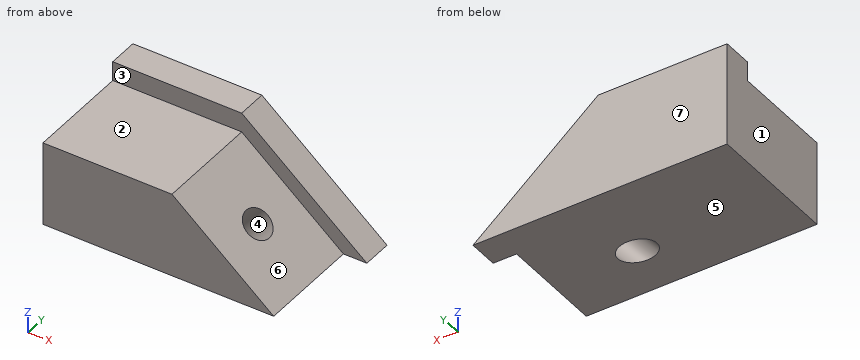
from build123d import *

# Parameters (mm, degrees)
F0_W     = 126.0763704777
F0_H     = 65.8090934157
F1_DEPTH = 50.8
F3_DEPTH = 51.054
F5_DEPTH = 25.4
F6_R     = 7.3849812588
F7_DEPTH = 47.244


with BuildPart() as f1:
    # F0 (on Top) → F1 (new body)
    with BuildSketch(Plane.XY):
        Rectangle(F0_W, F0_H)
    extrude(amount=F1_DEPTH)

    # F2 (on face) → F3 (cut)
    with BuildSketch(Plane.XZ.offset(32.9045467079)):
        Polygon((63.0381852388, 50.8), (-63.0381852388, 50.8), (-63.0381852388, 41.2882640958), (0, 41.2882640958), (49.7114025056, 0), (63.0381852388, 0), align=None)
    extrude(amount=-F3_DEPTH, mode=Mode.SUBTRACT)

    # F4 (on face) → F5 (cut)
    with BuildSketch(Plane.XZ.offset(-18.1494532921)):
        Polygon((63.0381852388, 50.8), (0, 50.8), (61.1636091415, 0), (63.0381852388, 0), align=None)
    extrude(amount=-F5_DEPTH, mode=Mode.SUBTRACT)

    # F6 (on face) → F7 (cut)
    with BuildSketch(Plane(origin=(20.2933884067, 0, 24.433403084), x_dir=(0.7692697728, 0, -0.6389241087), z_dir=(0.6389241087, 0, 0.7692697728))):
        with Locations((5.9307059858, -7.3775467079)):
            Circle(F6_R)
    extrude(amount=-F7_DEPTH, mode=Mode.SUBTRACT)


solid = f1.part
Verification items for the finished model (mm, model axes). Face numbers are marked on the shaded views. A direction names the side the tool comes from. Round coordinates to 2 decimals unless told otherwise and drop trailing zeros. Loops run counter-clockwise (first coordinate to the right, second up) from the corner with the lowest first, then second, coordinate; pieces in that order, holes last. Notation, with made-up numbers: (-11, -16) - (42, -16) arc R24 ccw to (42, -3) - close; hole circle Ø8 at (88, 9.5). An arc over 180 degrees is marked (long way). Use a Markdown table: item, result. Add a question column.
1. Section check A-A, the plane x = -54. Record the boundary of the cut face in (y, z).
2. Release check for a two-part mould opening along Z. For the marked faces 4, 5, 6 and 7 record: released by +Z, released by -Z, zero draft, split by the parting line, or undercut.
3. Section check C-C, the plane z = 34. Record the boundary of the cut face in (x, y).
4. Gauge pin test, flat ends, axial feed: pin 1 (15.5 mm diameter, centred on x = -30.5, y = -8, fed in from +Z); pin 2 (6 mm diameter, centred on x = 39.5, y = 23, fed in from +Z). Record the tip position at first contact, or that the pin passes through.
5. Section check B-B, the plane y = 21. Record the boundary of the cut face in (x, z), plus the area to 3 significant figures.
6. Access from +Z, -Z, +X, -X, +Y, -Y to the whole of each face (thin tool, end or side, straight path). Record for the marked faces 1, 2 and 3.
7. Section check D-D, the plane y = 13. Record the boundary of the cut face in (x, z), plus the area to 3 significant figures.
8. Thickness scan on probe 1 along Z at (x, y) = (-25, 18); probe 2 along Y at (x, z) = (-34, 48); probe 3 along X at (y, z) = (-11.5, 15.5). Record the ranges inside material, lowest first. Write a range as [from, to].
Checks:
| question | item | result |
|---|---|---|
| 1 | outline | (-32.9, 0) - (32.9, 0) - (32.9, 50.8) - (18.15, 50.8) - (18.15, 41.29) - (-32.9, 41.29) - close |
| 2 | face 4 | undercut |
| 2 | face 5 | released by -Z |
| 2 | face 6 | released by +Z |
| 2 | face 7 | zero draft |
| 3 | outline | (-63.04, -32.9) - (8.78, -32.9) - (8.78, 18.15) - (20.23, 18.15) - (20.23, 32.9) - (-63.04, 32.9) - close |
| 4 | pin 1 | stops at z = 41.29 |
| 4 | pin 2 | stops at z = 20.48 |
| 5 | outline | (-63.04, 0) - (61.16, 0) - (0, 50.8) - (-63.04, 50.8) - close |
| 5 | area | 4,760 mm^2 |
| 6 | face 1 | +Z, -Z, -X, +Y, -Y |
| 6 | face 2 | +Z, +X, -X, -Y |
| 6 | face 3 | +Z, +X, -Y |
| 7 | outline | (-63.04, 0) - (49.71, 0) - (0, 41.29) - (-63.04, 41.29) - close |
| 7 | area | 3,630 mm^2 |
| 8 | probe 1 | z = [0, 41.29] |
| 8 | probe 2 | y = [18.15, 32.9] |
| 8 | probe 3 | x = [-63.04, 12.62], [28.55, 31.05] |
